The listing builds one solid part. Answer for the finished solid, in the listing's coordinates (mm). A direction names the side the tool comes from. Give positions to 0.01 mm unless a question says otherwise; leave off trailing zeros. Write each loop counter-clockwise with the first axis right and the second up, starting at its lowest first coordinate (ties: lowest second). Pieces come first, ordered by that corner, then holes.
```python
from build123d import *

# Parameters (mm, degrees)
F2_R = 5
F3_T = -1


with BuildPart() as f1:
    # F0 (on Front) → F1 (revolve)
    with BuildSketch(Plane.XZ):
        Polygon((0, 117.396138), (-25, 117.396138), (-27.432391, 43.610401), (-24.728384, 26.710369), (-15.602366, 14.880346), (-3.979215, 12.396138), (-3.930857, -82.543589), (-28.446393, -92.603862), (0, -92.603862), align=None)
    revolve(axis=Axis((0, 0, 12.396138), (0, 0, -1)))

    # F2
    f2_edges = [f1.edges().sort_by_distance(p)[0] for p in [
        (3.930857, 0, -82.543589),
        (3.979215, 0, 12.396138),
    ]]
    fillet(f2_edges, radius=F2_R)

    # F3
    f3_openings = [f1.faces().sort_by_distance(p)[0] for p in [
        (0, 0, 117.396138),
    ]]
    offset(amount=F3_T, openings=f3_openings)


solid = f1.part
```
Item 1: Which of the six approach directions +Z, -Z, +X, -X, +Y, -Y give full straight-line access (tool end or side, diameter ignored) to faces 1 (the face through (20.023, -15.353, 80.019)), 2 (the face through (-9.4, 22.3, 117.396)), 3 (the face through (-2.73, -1.13, -36.03))?
Conclusion:
face 1: none
face 2: +Z, +X, -X, +Y, -Y
face 3: +Z
Item 2: Consider probe 1 along Z at (x, y) = (2, -4); probe 2 along Z at (x, y) = (-3.5, 15); probe 3 along X at (y, z) = (16, 22.5). Determine where each line is inside the solid, lowest interval first.
Conclusion:
probe 1: z = -92.6 to -91.6, -83.2 to -81.45, 10.52 to 12.31
probe 2: z = -92.6 to -91.6, -88.33 to -87.25, 14.84 to 16.26
probe 3: x = -14.33 to -12.36, 12.36 to 14.33
Item 3: Each of these flat-tipped pins is pushed along its axis until it touches: P1, Ø8, axis at x = -19, z = 70, coming from the +Y side; P2, Ø1.5, axis at y = 11.5, z = 77.5, coming from the -X side; P3, Ø4, axis at x = 13, z = 95.5, coming from the -Y side. Where does it stop, or does it pass through?
Conclusion:
P1: stops at y = 21.93
P2: stops at x = -24.02
P3: stops at y = -23.25
Item 4: A cutting plane is placed at B-B, the plane y = 20. Count the separate pieces of the cut face and the enclosed holes in it, plus the area to 3 significant figures.
Conclusion:
separate pieces: 2
enclosed holes: 1
area: 404 mm2
Item 5: A cutting plane is placed at C-C, the plane z = -69. Give the vertices of the cut face in (x, y), plus the area to 3 significant figures.
Conclusion:
outline: circle Ø7.88 at (0, 0); hole circle Ø5.88 at (0, 0)
area: 21.6 mm2
Item 6: A cutting plane is placed at A-A, the plane z = 98. Give the vertices of the cut face in (x, y), plus the area to 3 significant figures.
Conclusion:
outline: circle Ø51.28 at (0, 0); hole circle Ø49.28 at (0, 0)
area: 158 mm2
Item 7: Determine the mould class of faces 4 (the face through (-13.687, 21.468, 31.287)), 5 (the face through (0, 0, -92.604)), 6 (the face through (12.268, -9.407, 16.332)) for opening direction Z: pulls with the +Z half, pulls with the -Z half, needs draft (parallel to the pull), parting line crosses it, or undercut.
Conclusion:
face 4: undercut
face 5: pulls with the -Z half
face 6: pulls with the +Z half
